Read the model definition and answer for the solid it produces. Units are mm, in the model's axes. A direction names the side the tool comes from. Coordinates: 2 decimals unless noted, no trailing zeros. Order: outer loops, then holes, each group sorted by start corner. A loop starts at its lowest first (then second) coordinate and runs counter-clockwise, first axis right, second up. Notation, with made-up numbers: (69.25, 76) - (97.25, 76) arc R20 cw to (97.25, 115) - close; hole circle Ø10 at (-17, 36). An arc over 180 degrees is marked (long way). Write item = value, one per line.
from build123d import *

# Parameters (mm, degrees)
F0_R         = 8
F1_DEPTH     = 10
F2_R         = 11
F3_DEPTH     = 9
F5_DEPTH     = 2
F7_DEPTH     = 3
F8_R         = 1.75
F9_DEPTH     = 19.501
F10_R        = 3
F11_DEPTH    = 3
F12_T1_DEPTH = 8


# Not quite as in the source:
# - a fillet or chamfer that OpenCascade refuses, or shapes differently, is made with other operations: its cross-section is extruded or revolved along the edge and cut away or added


with BuildPart() as f1:
    # F0 (on Top) → F1 (new body)
    with BuildSketch(Plane.XY):
        with BuildLine():
            ThreePointArc((3.7080992435, -1.5), (-4, 0), (3.7080992435, 1.5))
            Line((3.7080992435, 1.5), (12, 1.5))
            Line((12, 1.5), (12, 6.5))
            Line((12, 6.5), (0, 6.5))
            ThreePointArc((0, 6.5), (-3.6055512755, 5.4083269132), (-6, 2.5))
            Line((-6, 2.5), (-13.9926491778, 2.5))
            ThreePointArc((-13.9926491778, 2.5), (-39.75, 0), (-13.9926491778, -2.5))
            Line((-13.9926491778, -2.5), (-6, -2.5))
            ThreePointArc((-6, -2.5), (-3.6055512755, -5.4083269132), (0, -6.5))
            Line((0, -6.5), (12, -6.5))
            Line((12, -6.5), (12, -1.5))
            Line((12, -1.5), (3.7080992435, -1.5))
        make_face()
        with Locations((-26.75, 0)):
            Circle(F0_R, mode=Mode.SUBTRACT)
    extrude(amount=F1_DEPTH)

    # F2 (on face) → F3 (cut)
    with BuildSketch(Plane.XY.offset(10)):
        with Locations((-26.75, 0)):
            Circle(F2_R)
    extrude(amount=-F3_DEPTH, mode=Mode.SUBTRACT)

    # F4 (on face) → F5 (cut)
    with BuildSketch(Plane.XY.offset(10)):
        with BuildLine():
            Line((-6, 2.5), (-13.9926491778, 2.5))
            ThreePointArc((-13.9926491778, 2.5), (-39.75, 0), (-13.9926491778, -2.5))
            Line((-13.9926491778, -2.5), (-6, -2.5))
            ThreePointArc((-6, -2.5), (-6.5, 0), (-6, 2.5))
        make_face()
    extrude(amount=-F5_DEPTH, mode=Mode.SUBTRACT)

    # F6 (on face) → F7 (cut)
    with BuildSketch(Plane(origin=(0, 6.5, 0), x_dir=(-1, 0, 0), z_dir=(0, 1, 0))):
        Polygon((-10, 6.6454482672), (-10, 3.3545517328), (-7.15, 1.7091034656), (-4.3, 3.3545517328), (-4.3, 6.6454482672), (-7.15, 8.2908965344), align=None)
    extrude(amount=-F7_DEPTH, mode=Mode.SUBTRACT)

    # F8 (on face) → F9 (cut, through all)
    with BuildSketch(Plane(origin=(0, 6.5, 0), x_dir=(-1, 0, 0), z_dir=(0, 1, 0))):
        with Locations((-7.15, 5)):
            Circle(F8_R)
    extrude(amount=-F9_DEPTH, mode=Mode.SUBTRACT)

    # F10 (on face) → F11 (cut)
    with BuildSketch(Plane.XZ.offset(6.5)):
        with Locations((7.15, 5)):
            Circle(F10_R)
    extrude(amount=-F11_DEPTH, mode=Mode.SUBTRACT)

    # F12: fillet of radius 5 on 4 edges, made by hand

    # F12_s2 → F12_t1 (join)
    with BuildSketch(Plane.XY):
        with BuildLine():
            ThreePointArc((-8.7177978871, -2.5), (-6.6326537465, -2.9555337043), (-4.9274509797, -4.2391304348))
            ThreePointArc((-4.9274509797, -4.2391304348), (-5.5324894844, -3.4119730516), (-6, -2.5))
            Line((-6, -2.5), (-8.7177978871, -2.5))
        make_face()
        with BuildLine():
            ThreePointArc((-14.9322285425, -5.4166666667), (-13.0872404524, -3.2918729423), (-10.386931828, -2.5))
            Line((-10.386931828, -2.5), (-13.9926491778, -2.5))
            ThreePointArc((-13.9926491778, -2.5), (-14.3762012754, -3.9861140379), (-14.9322285425, -5.4166666667))
        make_face()
        with BuildLine():
            ThreePointArc((-10.386931828, 2.5), (-13.0872404524, 3.2918729423), (-14.9322285425, 5.4166666667))
            ThreePointArc((-14.9322285425, 5.4166666667), (-14.3762012754, 3.9861140379), (-13.9926491778, 2.5))
            Line((-13.9926491778, 2.5), (-10.386931828, 2.5))
        make_face()
        with BuildLine():
            ThreePointArc((-4.9274509797, 4.2391304348), (-6.6326537465, 2.9555337043), (-8.7177978871, 2.5))
            Line((-8.7177978871, 2.5), (-6, 2.5))
            ThreePointArc((-6, 2.5), (-5.5324894844, 3.4119730516), (-4.9274509797, 4.2391304348))
        make_face()
    extrude(amount=F12_T1_DEPTH)


solid = f1.part
1) The part is cut by section D-D (z = 7.5). Determine the outline of the cut face in (x, y).
Returned:
outline = (-14.93, -5.42) arc R5 cw to (-10.39, -2.5) - (-8.72, -2.5) arc R5 cw to (-4.93, -4.24) arc R6.5 ccw to (0, -6.5) - (5.49, -6.5) - (5.49, -3.5) - (8.81, -3.5) - (8.81, -6.5) - (12, -6.5) - (12, -1.5) - (3.71, -1.5) arc R4 cw (long way) to (3.71, 1.5) - (12, 1.5) - (12, 6.5) - (8.52, 6.5) - (8.52, 3.5) - (5.78, 3.5) - (5.78, 6.5) - (0, 6.5) arc R6.5 ccw to (-4.93, 4.24) arc R5 cw to (-8.72, 2.5) - (-10.39, 2.5) arc R5 cw to (-14.93, 5.42) arc R13 ccw (long way) to start; hole circle Ø22 at (-26.75, 0)
2) The part is cut by section A-A (z = 5). Count the separate pieces of the cut face and the enclosed holes in it, and give its area (3 significant figures).
Returned:
separate_pieces = 3
enclosed_holes = 1
area = 293 mm^2
3) For faces 5 (the face through (-10, 2.5, 4)), 6 (the face through (-16.589, -4.213, 4.549)), 7 (the face through (4.3, 5, 5)), determine the directions among +Z, -Z, +X, -X, +Y, -Y from which every point of the face is accessible in a straight line to the end or side of a thin tool.
Returned:
face_5 = +Z, -Z, +Y
face_6 = +Z
face_7 = +Y
4) Determine the mould class of faces 1 (the face through (-13.1, 3.3, 3.9)), 2 (the face through (9, -1.5, 4)), 3 (the face through (5.745, 5.021, 2.52)), 4 (the face through (-39.74, 0.49, 3.94)) for opening direction Y: pulls with the +Y half, pulls with the -Y half, needs draft (parallel to the pull), parting line crosses it, or undercut.
Returned:
face_1 = pulls with the +Y half
face_2 = undercut
face_3 = needs draft
face_4 = parting line crosses it
5) Flat-ended cylindrical pins translate along their axes: pin 1 Ø4 at (x, z) = (7.5, 6.5) entering from -Y; pin 2 Ø4 at (x, y) = (2.5, 4.5) entering from -Z; pin 3 Ø0.9 at (y, z) = (4.5, 5) entering from -X; pin 4 Ø0.5 at (x, z) = (-10, 2) entering from -Y. Find the tip coordinate at first contact, or state that the pin passes through.
Returned:
pin_1 = -6.5
pin_2 = 0
pin_3 = -39.1
pin_4 = -2.5
6) Straight lines are drawn through the part: line 1 along Z through (x, y) = (7.15, -2.15); line 2 along Y through (x, z) = (-26.75, 0.6); line 3 along Y through (x, z) = (9.5, 2). For each, find the intervals that lie inside material, in ascending order. Write a range as from..to.
Returned:
line_1 = 0..3.25, 6.75..10
line_2 = -13..-8, 8..13
line_3 = -6.5..-1.5, 1.5..6.5
7) The part is cut by section B-B (y = 0). Determine the outline of the cut face in (x, z), and give its area (3 significant figures).
Returned:
outline = (-39.75, 0) - (-34.75, 0) - (-34.75, 1) - (-37.75, 1) - (-37.75, 8) - (-39.75, 8) - close; (-18.75, 0) - (-4, 0) - (-4, 10) - (-6.5, 10) - (-6.5, 8) - (-15.75, 8) - (-15.75, 1) - (-18.75, 1) - close
area = 121 mm^2
8) The part is cut by section C-C (x = -26.75). Determine the outline of the cut face in (y, z).
Returned:
outline = (-13, 0) - (-8, 0) - (-8, 1) - (-11, 1) - (-11, 8) - (-13, 8) - close; (8, 0) - (13, 0) - (13, 8) - (11, 8) - (11, 1) - (8, 1) - close
